Source: three-view drawing plus pictorial views. Frame: mm from the lowest corner of the part. A direction names the side the tool comes from. Give positions to 0.01 mm unless a question says otherwise; leave off trailing zeros. Order: outer loops, then holes, each group sorted by start corner. A loop starts at its lowest first (then second) coordinate and runs counter-clockwise, first axis right, second up. Notation, with made-up numbers: (25.5, 44.5) - (64.5, 44.5) arc R15 ccw to (64.5, 59.5) - close; hole circle Ø3 at (-18.75, 4). An arc over 180 degrees is marked (long way). Use one line per item in the form item = value.
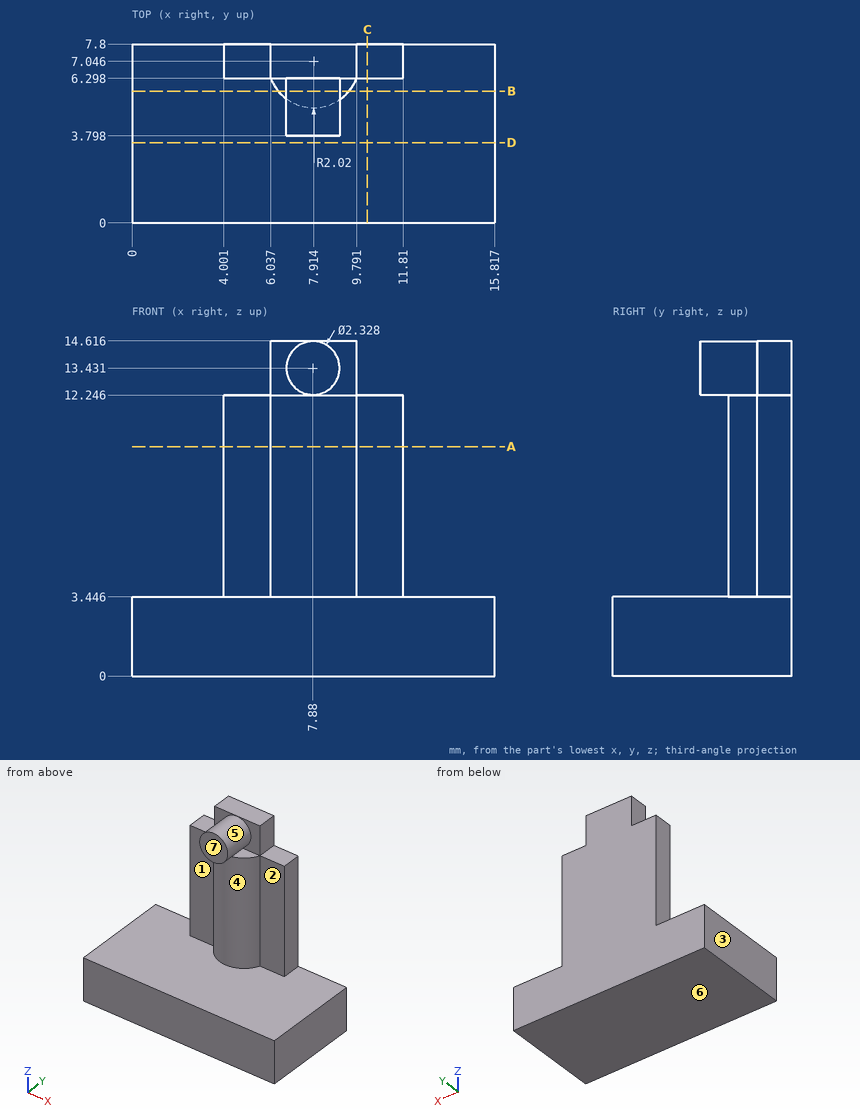
(1) Pull-direction query (Z, two-part tool) for the marked faces 4, 5, 6 and 7; classes: released by +Z, released by -Z, zero draft, split by the parting line, or undercut.
Computed values:
face_4 = undercut
face_5 = undercut
face_6 = released by -Z
face_7 = zero draft
(2) Reachability of the marked faces 1, 2 and 3 from +Z, -Z, +X, -X, +Y, -Y: full face, straight path, thin tool, end or side. Return the list, or none.
Computed values:
face_1 = +Z, -X, -Y
face_2 = +Z, +X, -Y
face_3 = +Z, -Z, -X, +Y, -Y
(3) Ray query, line 1 along Y through (x, z) = (5.75, 8); line 2 along Z through (x, y) = (10, 6.5) (1 decimal); line 3 along Y through (x, z) = (7.75, 13.5). Return the intervals inside material, ascending.
Computed values:
line_1 = 6.3 to 7.8
line_2 = 0 to 12.2
line_3 = 3.8 to 7.8
(4) Cut plane D-D on y = 3.5. Output: boundary loops of the cut face in (x, z) (1 decimal), plus the area to 3 significant figures.
Computed values:
outline = (0, 0) - (15.8, 0) - (15.8, 3.4) - (0, 3.4) - close
area = 54.5 mm²
(5) Cut plane A-A on z = 10. Output: boundary loops of the cut face in (x, y) (1 decimal), plus the area to 3 significant figures.
Computed values:
outline = (4, 6.3) - (6, 6.3) arc R2 ccw to (9.8, 6.3) - (11.8, 6.3) - (11.8, 7.8) - (4, 7.8) - close
area = 15.2 mm²
(6) Contact query for flat-ended pins moving along their axis: pin 1 Ø1.2 at (y, z) = (7.5, 13) entering from +X; pin 2 Ø4 at (x, z) = (3, 11) entering from -Y; pin 3 Ø0.7 at (x, z) = (8, 14) entering from -Y; pin 4 Ø1 at (x, z) = (13.5, 7.5) entering from -Y. Output: stop coordinate, or through.
Computed values:
pin_1 = 9.79
pin_2 = 6.3
pin_3 = 3.8
pin_4 = through
(7) Cut plane B-B on y = 5.75. Output: boundary loops of the cut face in (x, z) (1 decimal).
Computed values:
outline = (0, 0) - (15.8, 0) - (15.8, 3.4) - (9.5, 3.4) - (9.5, 12.2) - (6.4, 12.2) - (6.4, 3.4) - (0, 3.4) - close; circle Ø2.3 at (7.9, 13.4)
(8) Cut plane C-C on x = 10.25. Output: boundary loops of the cut face in (y, z) (1 decimal), plus the area to 3 significant figures.
Computed values:
outline = (0, 0) - (7.8, 0) - (7.8, 12.2) - (6.3, 12.2) - (6.3, 3.4) - (0, 3.4) - close
area = 40.1 mm²
